The figure shows three views and two pictorial views of one solid part (mm, origin at its lowest corner). Answer the questions. Give positions to 0.01 mm unless a question says otherwise; leave off trailing zeros. Loops run counter-clockwise (first coordinate to the right, second up) from the corner with the lowest first, then second, coordinate; pieces in that order, holes last. Notation, with made-up numbers: (-29, 39.5) - (30, 39.5) arc R23 cw to (30, 68.5) - close; hole circle Ø11 at (33.25, 45.5). An arc over 180 degrees is marked (long way). Use a Markdown table: item, result. Add a question column.
Item 1: A cutting plane is placed at B-B (x = 28). Determine the outline of the cut face in (y, z), plus the area to 3 significant figures.
Item 2: This flat-tipped pin is pushed along its axis until it touches: P1, Ø3, axis at x = 10.675, z = 45.325, coming from the +Y side. Where does it stop, or does it pass through?
Item 3: A cutting plane is placed at D-D (z = 51.5). Determine the outline of the cut face in (x, y), plus the area to 3 significant figures.
Item 4: Consider probe 1 along X at (y, z) = (2.35, 12); probe 2 along Z at (x, y) = (10.5, 0.65); probe 3 along Z at (x, y) = (10, 0.4). Determine where each line is inside the solid, lowest interval first. Write a range as [from, to].
Item 5: A cutting plane is placed at C-C (y = 2.25). Determine the outline of the cut face in (x, z) (1 decimal), plus the area to 3 significant figures.
Item 6: A cutting plane is placed at A-A (z = 28). Determine the outline of the cut face in (x, y).
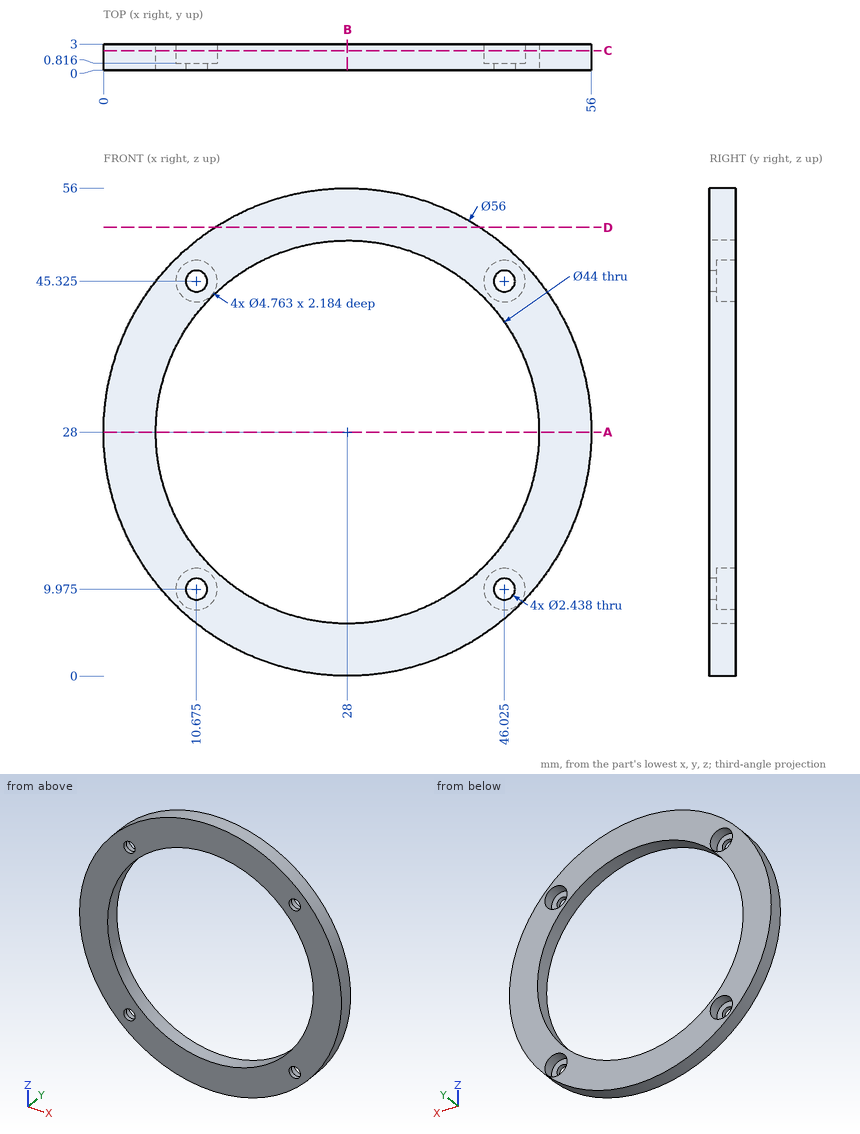
Geometry says:
| question | item | result |
|---|---|---|
| 1 | outline | (0, 0) - (3, 0) - (3, 6) - (0, 6) - close; (0, 50) - (3, 50) - (3, 56) - (0, 56) - close |
| 1 | area | 36.0 mm² |
| 2 | P1 | y = 0.82 |
| 3 | outline | (12.78, 0) - (43.22, 0) - (43.22, 3) - (12.78, 3) - close |
| 3 | area | 91.3 mm² |
| 4 | probe 1 | [5.02, 9.42], [11.93, 12.9], [43.1, 44.77], [47.28, 50.98] |
| 4 | probe 2 | [6.14, 8.77], [11.18, 14.67], [41.33, 44.12], [46.53, 49.86] |
| 4 | probe 3 | [6.55, 8.96], [10.99, 15.35], [40.65, 44.31], [46.34, 49.45] |
| 5 | outline | circle Ø56 at (28, 28); hole circle Ø44 at (28, 28); hole circle Ø4.8 at (10.7, 10); hole circle Ø4.8 at (10.7, 45.3); hole circle Ø4.8 at (46, 10); hole circle Ø4.8 at (46, 45.3) |
| 5 | area | 871 mm² |
| 6 | outline | (0, 0) - (6, 0) - (6, 3) - (0, 3) - close; (50, 0) - (56, 0) - (56, 3) - (50, 3) - close |
